Geometry: see drawing. Coordinates: mm, zero at the bounding-box minimum. Coordinates: 2 decimals unless noted, no trailing zeros. Loops run counter-clockwise (first coordinate to the right, second up) from the corner with the lowest first, then second, coordinate; pieces in that order, holes last. Notation, with made-up numbers: (18, 18.25) -> (31, 18.25) arc R25 ccw to (31, 45.25) -> close; hole circle Ø4 at (1.5, -18). An arc over 180 degrees is marked (long way). One line per item, written item: value. Start each with the question number.
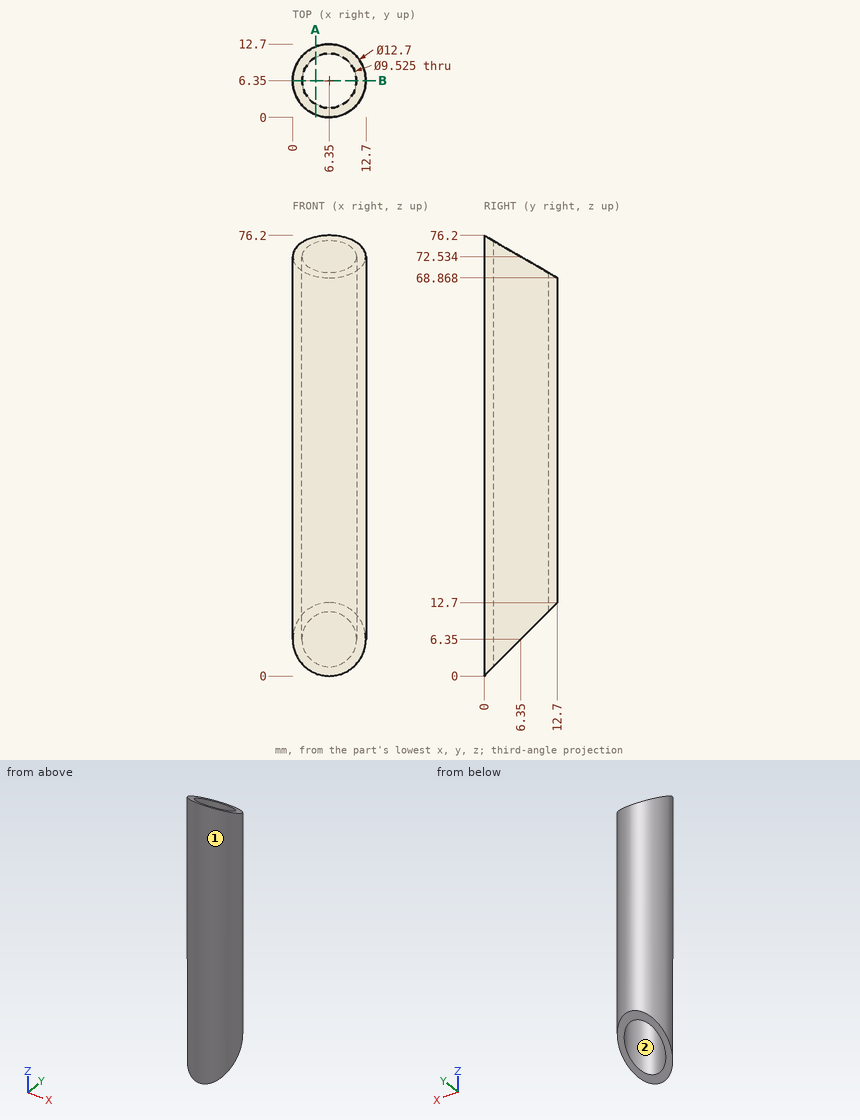
1. Draft query along Y for the marked faces 1 and 2. Return one class per face: released by +Y, released by -Y, zero draft, split by the parting line, or undercut.
2. Pin query (flat end, axial travel): pin 1 Ø2 at (x, z) = (9, 35) entering from -Y; pin 2 Ø1 at (x, z) = (10.5, 44) entering from -Y; pin 3 Ø1 at (x, z) = (3.5, 34) entering from +Y. Return the tip coordinate at first contact, or that it passes through.
3. Line query: L1, parallel to Y at x = 10.5, z = 33 (1 decimal); L2, parallel to X at y = 7.5, z = 27.5 (1 decimal); L3, parallel to Y at x = 7, z = 69.5 (1 decimal). Output: solid intervals per line, ascending. Write a range as [from, to].
4. Section A-A on x = 4. Return the cut outline in (y, z) (1 decimal).
5. Section B-B on y = 6.35. Return the cut outline in (x, z).
Checks:
1. face 1: split by the parting line
1. face 2: undercut
2. pin 1: y = 0.22
2. pin 2: y = 1.15
2. pin 3: y = 12.25
3. L1: [1.5, 4], [8.7, 11.2]
3. L2: [0.1, 1.7], [11, 12.6]
3. L3: [0, 1.6], [11.1, 11.6]
4. outline: (0.5, 0.5) -> (2.2, 2.2) -> (2.2, 74.9) -> (0.5, 75.9) -> close; (10.5, 10.5) -> (12.2, 12.2) -> (12.2, 69.1) -> (10.5, 70.1) -> close
5. outline: (0, 6.35) -> (1.59, 6.35) -> (1.59, 72.53) -> (0, 72.53) -> close; (11.11, 6.35) -> (12.7, 6.35) -> (12.7, 72.53) -> (11.11, 72.53) -> close
